For this review, take the finished solid that the model builds, in its own axes (mm). Round coordinates to 2 decimals unless told otherwise and drop trailing zeros. Order: outer loops, then holes, each group sorted by start corner. A loop starts at its lowest first (then second) coordinate and runs counter-clockwise, first axis right, second up. Notation, with made-up numbers: M 40,54 L 81,54 A24 ccw 81,70 Z; hole C -23.75,-24 d8. An arc over 180 degrees is marked long. Use a Markdown table: item, result.
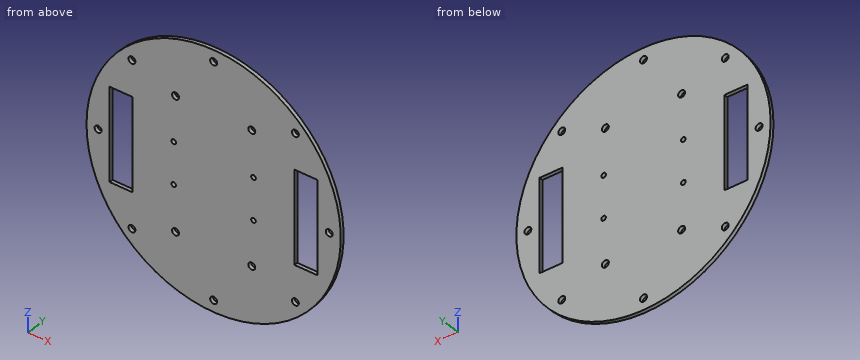
Autodesk Inventor part; units mm, degrees
ref_plane "YZ Plane" through (0, 0, 0) normal (1, 0, 0) x (0, 1, 0)
ref_plane "XZ Plane" through (0, 0, 0) normal (0, 1, 0) x (-1, 0, 0)
ref_plane "XY Plane" through (0, 0, 0) normal (0, 0, 1) x (1, 0, 0)
sketch "Эскиз1" plane through (0, 0, 0) normal (0, 1, 0) x (-1, 0, 0)
  circle A0 centre (0, 0) radius 55
  line L0 (79.4555, 0) -> (-79.4555, 0)
  line L1 (0, -103.8803) -> (0, 88.3129)
  dimension "d0" = 110
extrude "Выдавливание1" add sketch "Эскиз1" along normal blind 1.6
sketch "Эскиз2" plane through (0, 0, 0) normal (0, -1, 0) x (1, 0, 0)
  circle A0 centre (0, 0) radius 55
  line L0 (0, -103.8803) -> (0, 88.3129)
  line L1 (-79.4555, 0) -> (79.4555, 0)
  line L2 (11.5, -13.3) -> (23, -13.3)
  line L3 (23, -13.3) -> (23, 13.3)
  line L4 (23, 13.3) -> (11.5, 13.3)
  line L5 (11.5, 13.3) -> (11.5, -13.3)
  line L6 (35, -20) -> (45, -20)
  line L7 (45, -20) -> (45, 20)
  line L8 (45, 20) -> (35, 20)
  line L9 (35, 20) -> (35, -20)
  line L10 (17.25, -13.3) -> (17.25, 13.3)
  circle A1 centre (17.25, -9) radius 1
  circle A2 centre (17.25, 9) radius 1
  line L11 (3, 6) -> (33, 6)
  line L12 (33, 6) -> (33, -6)
  line L13 (33, -6) -> (3, -6)
  line L14 (3, -6) -> (3, 6)
  line L15 (-11.5, -13.3) -> (-23, -13.3)
  line L16 (-23, -13.3) -> (-23, 13.3)
  line L17 (-23, 13.3) -> (-11.5, 13.3)
  line L18 (-11.5, 13.3) -> (-11.5, -13.3)
  line L19 (-35, -20) -> (-45, -20)
  line L20 (-45, -20) -> (-45, 20)
  line L21 (-45, 20) -> (-35, 20)
  line L22 (-35, 20) -> (-35, -20)
  line L23 (-17.25, -13.3) -> (-17.25, 13.3)
  circle A3 centre (-17.25, -9) radius 1
  circle A4 centre (-17.25, 9) radius 1
  line L24 (-3, 6) -> (-33, 6)
  line L25 (-33, 6) -> (-33, -6)
  line L26 (-33, -6) -> (-3, -6)
  line L27 (-3, -6) -> (-3, 6)
  circle A5 centre (0, 0) radius 50
  circle A6 centre (0, -50) radius 1.5
  circle A7 centre (50, 0) radius 1.5
  circle A8 centre (0, 50) radius 1.5
  circle A9 centre (-50, 0) radius 1.5
  circle A10 centre (35.3553, -35.3553) radius 1.5
  circle A11 centre (50, 0) radius 1.5
  circle A12 centre (35.3553, 35.3553) radius 1.5
  circle A13 centre (0, 50) radius 1.5
  circle A14 centre (-35.3553, 35.3553) radius 1.5
  circle A15 centre (-50, 0) radius 1.5
  circle A16 centre (-35.3553, -35.3553) radius 1.5
  dimension "d6" = 11.5
  dimension "d7" = 26.6
  dimension "d9" = 10
  dimension "d10" = 40
  dimension "d11" = 45
  dimension "d12" = 12
  dimension "d13" = 2
  dimension "d14" = 18
  dimension "d15" = 2
  dimension "d16" = 30
  dimension "d17" = 12
  dimension "d18" = 2
  dimension "d21" = 100
  dimension "d22" = 3
  dimension "d23" = 3
  dimension "d25" = 3
  dimension "d26" = 3
  dimension "d30" = 360
extrude "Выдавливание2" cut sketch "Эскиз2" against normal blind 1.6 contours A7 A5 L1 | L1 A5 A7 | A8 A5 L0 | L0 A5 A8 | A6 A5 L0 | L0 A5 A6 | A5 A7 L1 | L1 A7 A5 | A9 A5 L1 | L1 A5 A9 | A5 A8 L0 | L0 A8 A5 | A5 A6 L0 | L0 A6 A5 | A12 A5 | A5 A12 | A10 A5 | A5 A10 | A5 A9 L1 | L1 A9 A5 | A14 A5 | A5 A14 | A16 A5 | A5 A16 | L7 L6 L9 L1 | L1 L9 L8 L7 | L20 L21 L22 L1 | L1 L22 L19 L20 | A3 L23 | L23 A3 | A4 L23 | L23 A4 | A1 L10 | L10 A1 | A2 L10 | L10 A2
sketch "Эскиз3" plane through (0, 0, 0) normal (0, -1, 0) x (1, 0, 0)
  circle A0 centre (50, 0) radius 1.5
  circle A1 centre (-50, 0) radius 1.5
  circle A2 centre (-17.25, 9) radius 1
  line L0 (35, -20) -> (35, 20)
  line L1 (35, 20) -> (45, 20)
  line L2 (45, 20) -> (45, -20)
  line L3 (45, -20) -> (35, -20)
  line L4 (-35, -20) -> (-45, -20)
  line L5 (-45, -20) -> (-45, 20)
  line L6 (-45, 20) -> (-35, 20)
  line L7 (-35, 20) -> (-35, -20)
  circle A3 centre (-35.3553, 35.3553) radius 1.5
  circle A4 centre (35.3553, -35.3553) radius 1.5
  circle A5 centre (35.3553, 35.3553) radius 1.5
  circle A6 centre (-35.3553, -35.3553) radius 1.5
  circle A7 centre (17.25, 9) radius 1
  circle A8 centre (17.25, -9) radius 1
  circle A9 centre (-17.25, -9) radius 1
  circle A10 centre (0, 50) radius 1.5
  circle A11 centre (0, -50) radius 1.5
  circle A12 centre (0, 0) radius 55
  line L8 (-79.4555, 0) -> (79.4555, 0)
  line L9 (0, -103.8803) -> (0, 88.3129)
  circle A13 centre (0, 0) radius 50
  circle A14 centre (-35.3553, -35.3553) radius 1.5
  line L10 (23, 13.3) -> (11.5, 13.3)
  line L11 (-21.1, -39.0646) -> (21.1, -39.0646)
  line L12 (21.1, -39.0646) -> (21.1, 37.2354)
  line L13 (21.1, 37.2354) -> (-21.1, 37.2354)
  line L14 (-21.1, 37.2354) -> (-21.1, -39.0646)
  circle A15 centre (-16.5, -28.5) radius 1.5
  circle A16 centre (16.5, -28.5) radius 1.5
  circle A17 centre (16.5, 28.5) radius 1.5
  circle A18 centre (-16.5, 28.5) radius 1.5
  dimension "d34" = 76.3
  dimension "d35" = 42.2
  dimension "d37" = 3
  dimension "d38" = 3
  dimension "d39" = 3
  dimension "d40" = 3
  dimension "d42" = 33
  dimension "d43" = 57
extrude "Выдавливание3" cut sketch "Эскиз3" against normal blind 1.6 contours A15 | A16 | A17 | A18
properties part number "pcbCase"
Q1. Add section D-D (z = -50). Write out the cut boundary in (x, y).
Determined:
| item | result |
|---|---|
| outline | M -22.91,0 L -1.5,0 L -1.5,1.6 L -22.91,1.6 Z; M 1.5,0 L 22.91,0 L 22.91,1.6 L 1.5,1.6 Z |
Q2. Add section A-A (z = 0). Write out the cut boundary in (x, y), then the cut area to 3 significant figures.
Determined:
| item | result |
|---|---|
| outline | M -55,0 L -51.5,0 L -51.5,1.6 L -55,1.6 Z; M -48.5,0 L -45,0 L -45,1.6 L -48.5,1.6 Z; M -35,0 L 35,0 L 35,1.6 L -35,1.6 Z; M 45,0 L 48.5,0 L 48.5,1.6 L 45,1.6 Z; M 51.5,0 L 55,0 L 55,1.6 L 51.5,1.6 Z |
| area | 134 mm^2 |
Q3. Add section B-B (x = 0). Write out the cut boundary in (y, z), then the cut area to 3 significant figures.
Determined:
| item | result |
|---|---|
| outline | M 0,-55 L 1.6,-55 L 1.6,-51.5 L 0,-51.5 Z; M 0,-48.5 L 1.6,-48.5 L 1.6,48.5 L 0,48.5 Z; M 0,51.5 L 1.6,51.5 L 1.6,55 L 0,55 Z |
| area | 166 mm^2 |
Q4. Wall thickness on line 1 along Z through (x, y) = (0, 0.3); line 2 along Z through (x, y) = (-17.25, 0.55); line 3 along Z through (x, y) = (-16.5, 1.1): over which ranges is each line inside the solid? List them lowest first. Write a range as [from, to].
Determined:
| item | result |
|---|---|
| line 1 | z = [-55, -51.5], [-48.5, 48.5], [51.5, 55] |
| line 2 | z = [-52.22, -29.8], [-27.2, -10], [-8, 8], [10, 27.2], [29.8, 52.22] |
| line 3 | z = [-52.47, -30], [-27, -9.66], [-8.34, 8.34], [9.66, 27], [30, 52.47] |
Q5. Clearance check with flat-ended pins moving along their axes: pin 1 (1.8 mm diameter, centred on x = -17.25, z = -9, fed in from -Y); pin 2 (0.8 mm diameter, centred on y = 1, z = -1, fed in from +X); pin 3 (0.5 mm diameter, centred on x = -40.5, y = 1, fed in from +Z). State where each tip first meets the part, or that it passes through.
Determined:
| item | result |
|---|---|
| pin 1 | passes through |
| pin 2 | stops at x = 55 |
| pin 3 | stops at z = 37.48 |
Q6. Add section C-C (z = -15.5). Write out the cut boundary in (x, y), then the cut area to 3 significant figures.
Determined:
| item | result |
|---|---|
| outline | M -52.77,0 L -45,0 L -45,1.6 L -52.77,1.6 Z; M -35,0 L 35,0 L 35,1.6 L -35,1.6 Z; M 45,0 L 52.77,0 L 52.77,1.6 L 45,1.6 Z |
| area | 137 mm^2 |
